from build123d import *

# Parameters (mm, degrees)
SKETCH_1_R               = 21.8
SKETCH_1_R_2             = 4
EXTRUDE_1_DEPTH          = 10
SKETCH_2_R               = 12.5
SKETCH_2_R_2             = 4
EXTRUDE_2_DEPTH          = 6
CUT_EXTRUDE_1_REACH      = 36.734
CUT_EXTRUDE_1_END_RADIUS = 12.5
SKETCH_3_R               = 1


with BuildPart() as part:
    # 草圖1 → 填料-伸長1 (new body)
    with BuildSketch(Plane(origin=(0, 0, 0), x_dir=(1, 0, 0), z_dir=(0, 1, 0))):
        with Locations(Location((0, 0, 0), (0, 0, 270))):
            Circle(SKETCH_1_R)
        with Locations(Location((0, 0, 0), (0, 0, 270))):
            Circle(SKETCH_1_R_2, mode=Mode.SUBTRACT)
    extrude(amount=EXTRUDE_1_DEPTH)

    # 草圖2 → 填料-伸長2 (add)
    with BuildSketch(Plane(origin=(0, 10, 0), x_dir=(1, 0, 0), z_dir=(0, 1, 0))):
        with Locations(Location((0, 0, 0), (0, 0, 270))):
            Circle(SKETCH_2_R)
        with Locations(Location((0, 0, 0), (0, 0, 270))):
            Circle(SKETCH_2_R_2, mode=Mode.SUBTRACT)
    extrude(amount=EXTRUDE_2_DEPTH)

    # 除料-伸長1: up to this cylinder (the profile starts inside it)
    cut_extrude_1_end = Plane(origin=(0, 13, 0), z_dir=(0, -1, 0)) * Cylinder(CUT_EXTRUDE_1_END_RADIUS, 99.468, mode=Mode.PRIVATE)
    # 草圖3 → 除料-伸長1 (cut, up to the surface)
    with BuildSketch(Plane.XY, mode=Mode.PRIVATE) as cut_extrude_1_sk1:
        with Locations(Location((0, 13, 0), (0, 0, 180))):
            Circle(SKETCH_3_R)
    cut_extrude_1_tool1 = extrude(cut_extrude_1_sk1.sketch, amount=CUT_EXTRUDE_1_REACH, mode=Mode.PRIVATE) & cut_extrude_1_end
    add(cut_extrude_1_tool1.solids().sort_by_distance((0, 13, 0))[0], mode=Mode.SUBTRACT)


solid = part.part
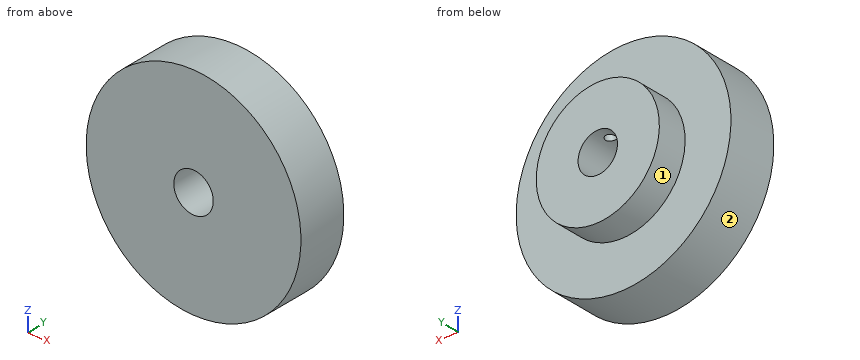
Geometry: final body of the model. Coordinates: model frame, mm. Face numbers are marked on the shaded views. A direction names the side the tool comes from. Round coordinates to 2 decimals unless told otherwise and drop trailing zeros. Order: outer loops, then holes, each group sorted by start corner. A loop starts at its lowest first (then second) coordinate and runs counter-clockwise, first axis right, second up.
Q1. Section B-B, the plane z = 0. Output: boundary loops of the cut face in (x, y).
Result sheet:
outline: (-21.8, 0) - (-4, 0) - (-4, 16) - (-12.5, 16) - (-12.5, 10) - (-21.8, 10) - close; (4, 0) - (21.8, 0) - (21.8, 10) - (12.5, 10) - (12.5, 16) - (4, 16) - close
Q2. Pin query (flat end, axial travel): pin 1 (12 mm diameter, centred on x = 11.5, z = -16.5, fed in from +Y); pin 2 (8 mm diameter, centred on y = 2, z = 9.5, fed in from +X); pin 3 (2.5 mm diameter, centred on x = 0, y = 13, fed in from +Z). Return the tip coordinate at first contact, or that it passes through.
Result sheet:
pin 1: stops at y = 10
pin 2: stops at x = 21.09
pin 3: stops at z = 12.5
Q3. Section A-A, the plane x = 0. Output: boundary loops of the cut face in (y, z).
Result sheet:
outline: (0, -21.8) - (10, -21.8) - (10, -12.5) - (16, -12.5) - (16, -4) - (0, -4) - close; (0, 4) - (12, 4) - (12, 12.5) - (10, 12.5) - (10, 21.8) - (0, 21.8) - close; (14, 4) - (16, 4) - (16, 12.5) - (14, 12.5) - close
Q4. Material intervals for probe 1 along X at (y, z) = (10.25, 0); probe 2 along X at (y, z) = (9.25, 0); probe 3 along Y at (x, z) = (0, 9), sorted ascending.
Result sheet:
probe 1: x = -12.5 to -4, 4 to 12.5
probe 2: x = -21.8 to -4, 4 to 21.8
probe 3: y = 0 to 12, 14 to 16
Q5. Section C-C, the plane y = 4.75. Output: boundary loops of the cut face in (x, z), and give its area (3 significant figures).
Result sheet:
outline: circle Ø43.6 at (0, 0); hole circle Ø8 at (0, 0)
area: 1,440 mm2
Q6. Access query for the marked faces 1 and 2. Directions: +Z, -Z, +X, -X, +Y, -Y. A direction counts if a zero-diameter tool reaches every point of the face in a straight line with its end or side. Return the directions, or none.
Result sheet:
face 1: +Y
face 2: +Y, -Y
Q7. Section D-D, the plane z = 11. Output: boundary loops of the cut face in (x, y).
Result sheet:
outline: (-18.82, 0) - (18.82, 0) - (18.82, 10) - (5.94, 10) - (5.94, 16) - (-5.94, 16) - (-5.94, 10) - (-18.82, 10) - close; hole circle Ø2 at (0, 13)
